from build123d import *

# Parameters (mm, degrees)
SKETCH1_R           = 1.575
BOSS_EXTRUDE1_DEPTH = 5
SKETCH2_R           = 4.88448764
CUT_EXTRUDE1_DEPTH  = 2.5


with BuildPart() as part:
    # Sketch1 → Boss-Extrude1 (new, symmetric)
    with BuildSketch(Plane.XY):
        with BuildLine():
            Line((1.186113957, -2.83703343), (-0.446593535, -3.519639818))
            ThreePointArc((-0.446593535, -3.519639818), (-1.640687739, -4.995254909), (-1.064164547, -6.803823921))
            ThreePointArc((-1.064164547, -6.803823921), (-2.49573113, -12.009536189), (-6.097709737, -7.987773738))
            Line((-6.097709737, -7.987773738), (-2.8979158, 1.028449811))
            ThreePointArc((-2.8979158, 1.028449811), (2.113777793, 2.233286466), (1.186113957, -2.83703343))
        make_face()
        Circle(SKETCH1_R, mode=Mode.SUBTRACT)
        with Locations((-3.199793936, -9.016223549)):
            Circle(SKETCH1_R, mode=Mode.SUBTRACT)
    extrude(amount=BOSS_EXTRUDE1_DEPTH, both=True)

    # Sketch2 → Cut-Extrude1 (cut)
    with BuildSketch(Plane.XY.offset(5)):
        with Locations((-3.199793936, -9.016223549)):
            Circle(SKETCH2_R)
    cut_extrude1 = extrude(amount=-CUT_EXTRUDE1_DEPTH, mode=Mode.SUBTRACT)

    # Mirror1: Cut-Extrude1 across plane
    add(cut_extrude1.mirror(Plane.XY), mode=Mode.SUBTRACT)


solid = part.part
Verification items for the finished model (mm, model axes). A direction names the side the tool comes from. Give positions to 0.01 mm unless a question says otherwise; leave off trailing zeros. Write each loop counter-clockwise with the first axis right and the second up, starting at its lowest first coordinate (ties: lowest second). Pieces come first, ordered by that corner, then holes.
(1) Access from +Z, -Z, +X, -X, +Y, -Y to the whole of each face (thin tool, end or side, straight path). Record for faces 5 (the face through (-3.114, -4.132, 3.768)), 6 (the face through (-1.25, -0.96, -0.07)).
(2) Cross-section at A-A (y = -10). Enter the section's corners in (x, z).
(3) Cross-section at D-D (y = 0.25). Enter the section's corners in (x, z), plus the area to 3 significant figures.
(4) Material ranges on line 1 (Z direction, x = -5.25, y = -11); line 2 (Y direction, x = -0.5, z = -4); line 3 (Y direction, x = 0, z = -1) (3 decimals), recorded low to high.
(5) Mould release check, pull along X, two halves, no side actions. Record for faces 1 (the face through (-2, -1, -5)), 2 (the face through (-3.114, -4.132, -3.768)), 3 (the face through (2.05, 2.29, 0.07)), 4 (the face through (0.381, -3.174, 0.07)): +X half, -X half, draft (parallel to the pull), parting line (faces both ways), or undercut.
(6) Cross-section at C-C (z = 3). Enter the section's corners in (x, y) (3 decimals).
(7) Cross-section at B-B (z = -1.5). Enter the section's corners in (x, y) (3 decimals), plus the area to 3 significant figures.
(8) Gauge pin test, flat ends, axial feed: pin 1 (2.5 mm diameter, centred on x = -3.2, y = -9.02, fed in from +Z); pin 2 (1.5 mm diameter, centred on y = -10, z = -1, fed in from -X); pin 3 (4 mm diameter, centred on y = 0.5, z = 1.5, fed in from -X); pin 4 (5 mm diameter, centred on x = -4.5, y = -8, fed in from -Z). Record the tip position at first contact, or that the pin passes through.
Worked out:
1. face 5: +Z, -Y
1. face 6: +Z, -Z
2. outline: (-6.11, -2.5) - (-4.43, -2.5) - (-4.43, 2.5) - (-6.11, 2.5) - close; (-1.97, -2.5) - (-0.29, -2.5) - (-0.29, 2.5) - (-1.97, 2.5) - close
3. outline: (-3.17, -5) - (-1.56, -5) - (-1.56, 5) - (-3.17, 5) - close; (1.56, -5) - (3.06, -5) - (3.06, 5) - (1.56, 5) - close
3. area: 31.3 mm2
4. line 1: z = -2.5 to 2.5
4. line 2: y = -3.54 to -1.49, 1.49 to 3.03
4. line 3: y = -3.333 to -1.575, 1.575 to 3.075
5. face 1: draft
5. face 2: undercut
5. face 3: parting line
5. face 4: +X half
6. outline: (-4.828, -4.411) arc R4.884 cw to (-1.456, -4.454) arc R2 cw to (-0.447, -3.52) - (1.186, -2.837) arc R3.075 ccw (long way) to (-2.898, 1.028) - close; hole circle Ø3.15 at (0, 0)
7. outline: (-6.098, -7.988) arc R3.075 ccw (long way) to (-1.064, -6.804) arc R2 cw to (-0.447, -3.52) - (1.186, -2.837) arc R3.075 ccw (long way) to (-2.898, 1.028) - close; hole circle Ø3.15 at (-3.2, -9.016); hole circle Ø3.15 at (0, 0)
7. area: 59.9 mm2
8. pin 1: passes through
8. pin 2: stops at x = -6.27
8. pin 3: stops at x = -3.8
8. pin 4: stops at z = -2.5
